```python
from build123d import *

# Parameters (mm, degrees)
F0_R     = 1.905
F1_DEPTH = 5


with BuildPart() as f1:
    # F0 (on Front) → F1 (new body)
    with BuildSketch(Plane.XZ):
        with BuildLine():
            Line((65.113842, 89.450538), (19.638577, 89.450538))
            Line((19.638577, 89.450538), (19.638577, 79.722829))
            Line((19.638577, 79.722829), (14.755342, 79.722829))
            Line((14.755342, 79.722829), (2.940716, 69.650203))
            ThreePointArc((2.940716, 69.650203), (1.762344, 68.177362), (1.214478, 66.372462))
            Line((1.214478, 66.372462), (1.214478, 49.523853))
            ThreePointArc((1.214478, 49.523853), (1.301303, 48.742133), (1.557545, 47.998518))
            Line((1.557545, 47.998518), (22.394331, 6.778323))
            ThreePointArc((22.394331, 6.778323), (25.894047, 3.30378), (30.777479, 2.616351))
            Line((30.777479, 2.616351), (68.54441, 11.307366))
            ThreePointArc((68.54441, 11.307366), (82.783914, 21.945088), (84.528677, 39.633512))
            Line((84.528677, 39.633512), (69.979429, 79.702094))
            Line((69.979429, 79.702094), (65.113842, 79.702094))
            Line((65.113842, 79.702094), (65.113842, 89.450538))
        make_face()
        with Locations((28.860504, 9.454119)):
            Circle(F0_R, mode=Mode.SUBTRACT)
        with Locations((71.314917, 21.167528)):
            Circle(F0_R, mode=Mode.SUBTRACT)
        Polygon((65.114856, 19.524755), (32.888938, 42.093192), (44.271119, 58.196455), (76.398229, 35.488227), align=None, mode=Mode.SUBTRACT)
        with Locations((77.09127, 29.339786)):
            Circle(F0_R, mode=Mode.SUBTRACT)
        with Locations((6.189452, 53.549591)):
            Circle(F0_R, mode=Mode.SUBTRACT)
        with Locations((6.192373, 63.382605)):
            Circle(F0_R, mode=Mode.SUBTRACT)
        with Locations((32.347996, 48.456819)):
            Circle(F0_R, mode=Mode.SUBTRACT)
        with Locations((38.124348, 56.629078)):
            Circle(F0_R, mode=Mode.SUBTRACT)
        with Locations((25.618793, 84.67719)):
            Circle(F0_R, mode=Mode.SUBTRACT)
        with Locations((63.986167, 59.999965)):
            Circle(F0_R, mode=Mode.SUBTRACT)
        with Locations((59.080809, 84.597848)):
            Circle(F0_R, mode=Mode.SUBTRACT)
    extrude(amount=-F1_DEPTH)


solid = f1.part
```
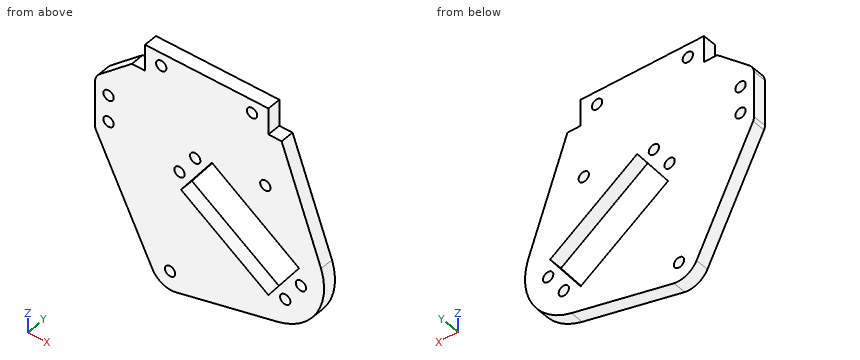
For this review, take the finished solid that the model builds, in its own axes (mm). Give positions to 0.01 mm unless a question says otherwise; leave off trailing zeros. Write each loop counter-clockwise with the first axis right and the second up, starting at its lowest first coordinate (ties: lowest second). Pieces come first, ordered by that corner, then holes. Notation, with made-up numbers: M 2.25,49 L 37.25,49 A25 cw 37.25,72 Z; hole C 51,-16 d3. An arc over 180 degrees is marked long. One line per item, written item: value.
1) Take a section at C-C, the plane x = 56. Write out the cut boundary in (y, z).
Results are:
outline: M 0,8.42 L 5,8.42 L 5,25.91 L 0,25.91 Z; M 0,49.91 L 5,49.91 L 5,89.45 L 0,89.45 Z
2) Take a section at B-B, the plane z = 41. Write out the cut boundary in (x, y).
Results are:
outline: M 5.1,0 L 34.45,0 L 34.45,5 L 5.1,5 Z; M 68.6,0 L 84.03,0 L 84.03,5 L 68.6,5 Z
3) Take a section at A-A, the plane x = 38.5. Write out the cut boundary in (y, z).
Results are:
outline: M 0,4.39 L 5,4.39 L 5,38.16 L 0,38.16 Z; M 0,50.03 L 5,50.03 L 5,54.76 L 0,54.76 Z; M 0,58.5 L 5,58.5 L 5,89.45 L 0,89.45 Z
4) For line 1 (X direction, y = 1.9, z = 29); line 2 (X direction, y = 4, z = 21.5); line 3 (Z direction, x = 63, y = 4.7), list the stretches that pass through material, from the lowest coordinate up. Write a range as from..to.
Results are:
line 1: x = 11.16..51.58, 71.81..75.22, 78.97..85.3
line 2: x = 14.95..62.29, 66.51..69.44, 73.19..82.53
line 3: z = 10.03..21.01, 44.96..58.37, 61.63..89.45
5) For P1, Ø3.5, axis at x = 63.99, z = 60, coming from the -Y side; P2, Ø2, axis at x = 53, y = 2.5, coming from the -Z side; P3, Ø2.5, axis at x = 17, y = 2.5, coming from the +Z side; P4, Ø2, axis at x = 62, y = 2, coming from the -Z side, all flat-tipped, find the tip position at first contact; note any pin that passes through.
Results are:
P1: passes through
P2: stops at z = 7.5
P3: stops at z = 79.72
P4: stops at z = 9.57
6) Take a section at D-D, the plane y = 2.45. Count the separate pieces of the cut face and the enclosed holes in it, then the cut area to 3 significant figures.
Results are:
separate pieces: 1
enclosed holes: 11
area: 4,700 mm²
